```python
from build123d import *

# Parameters (mm, degrees)
SKETCH_18_R = 2


with BuildPart() as part:
    # ｽｲｰﾌﾟ6: sweep along a path in ｽｹｯﾁ19
    with BuildLine(Plane.XY) as sweep_6_path:
        Line((0, 0), (0, 26))
        ThreePointArc((0, 26), (2.343145751, 31.656854249), (8, 34))
        Line((8, 34), (26, 34))
        ThreePointArc((26, 34), (31.656854249, 36.343145751), (34, 42))
        Line((34, 42), (34, 68))
    # ｽｹｯﾁ18 → ｽｲｰﾌﾟ6 (sweep)
    with BuildSketch(Plane(origin=(0, 0, 0), x_dir=(1, 0, 0), z_dir=(0, 1, 0))):
        Circle(SKETCH_18_R)
    sweep(path=sweep_6_path.line)


solid = part.part
```
For this review, take the finished solid that the model builds, in its own axes (mm). A direction names the side the tool comes from. Coordinates: 2 decimals unless noted, no trailing zeros. Order: outer loops, then holes, each group sorted by start corner. A loop starts at its lowest first (then second) coordinate and runs counter-clockwise, first axis right, second up. Notation, with made-up numbers: (-31, -29.5) -> (-6, -29.5) arc R17 cw to (-6, -10.5) -> close; hole circle Ø1 at (-8, -18). An arc over 180 degrees is marked (long way). Use CSV: the item, a comma, the result in double quotes. Start each with the question number.
Item 1: We need section B-B, the plane x = 23.5. Give the boundary of the cut face in (y, z), then the cut area to 3 significant figures.
Item 2: Wall thickness on probe 1 along Y at (x, z) = (12, 0.1); probe 2 along X at (y, z) = (23, 0.6); probe 3 along X at (y, z) = (51, -0.55): over which ranges is each line inside the solid? List them lowest first.
Item 3: For faces 1 (the face through (0, 13, 2)), 2 (the face through (17.126, 32.153, 0.766)), 3 (the face through (34, 68, 0)), 4 (the face through (35.847, 55.182, 0.766)), list the 3-axis set-ups (+Z, -Z, +X, -X, +Y, -Y) from which the entire face can be reached by the end or side of a thin tool; tool diameter is ignored.
Item 4: Insertion check: pin 1 (1 mm diameter, centred on y = 45.5, z = 0.5, fed in from -X). The pin has a flat end and moves straight along its axis. Give the tip position at first contact, or say it passes through.
Item 5: We need section A-A, the plane z = 0. Give the boundary of the cut face in (x, y), then the cut area to 3 significant figures.
Derived:
1,outline,"circle Ø4 at (34, 0)"
1,area,"12.6 mm^2"
2,probe 1,"y = 32 to 36"
2,probe 2,"x = -1.91 to 1.91"
2,probe 3,"x = 32.08 to 35.92"
3,face 1,"-Y"
3,face 2,"none"
3,face 3,"+Z, -Z, +X, -X, +Y"
3,face 4,"+Y"
4,pin 1,"stops at x = 32"
5,outline,"(-2, 0) -> (2, 0) -> (2, 26) arc R6 cw to (8, 32) -> (26, 32) arc R10 ccw to (36, 42) -> (36, 68) -> (32, 68) -> (32, 42) arc R6 cw to (26, 36) -> (8, 36) arc R10 ccw to (-2, 26) -> close"
5,area,"381 mm^2"
